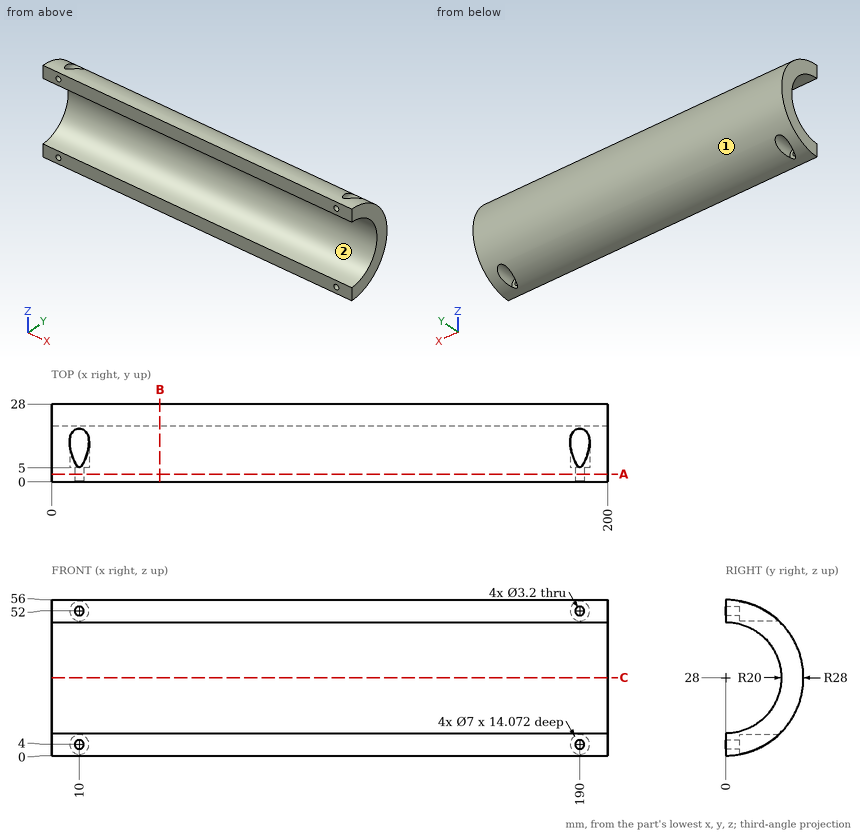
Answer from the drawing. Dimensions are ordinates in mm from the lowest x, y and z of the part. Give positions to 0.01 mm unless a question says otherwise; leave off trailing zeros. Loops run counter-clockwise (first coordinate to the right, second up) from the corner with the lowest first, then second, coordinate; pieces in that order, holes last. Notation, with made-up numbers: (9.25, 17) - (58.25, 17) arc R22 ccw to (58.25, 37) - close; hole circle Ø7 at (37.5, 2.25). An arc over 180 degrees is marked (long way). Answer as a JSON object with one key per item and string values.
1. Flat-ended cylindrical pins translate along their axes: pin 1 Ø2 at (x, z) = (11, 53) entering from +Y; pin 2 Ø11 at (x, z) = (190, 4) entering from +Y; pin 3 Ø1 at (x, z) = (102.5, 21.5) entering from +Y. Find the tip coordinate at first contact, or state that the pin passes through.
Determined:
{"pin 1": "y = 5", "pin 2": "y = 21.02", "pin 3": "y = 27.35"}
2. A cutting plane is placed at B-B (x = 39). Write down the section's boundary in (y, z).
Determined:
{"outline": "(0, 0) arc R28 ccw to (0, 56) - (0, 48) arc R20 cw to (0, 8) - close"}
3. A cutting plane is placed at A-A (y = 2.75). Write down the section's boundary in (x, z) (1 decimal), then the cut area to 3 significant figures.
Determined:
{"outline": "(0, 0.1) - (200, 0.1) - (200, 8.2) - (0, 8.2) - close; (0, 47.8) - (200, 47.8) - (200, 55.9) - (0, 55.9) - close; hole circle Ø3.2 at (10, 4); hole circle Ø3.2 at (10, 52); hole circle Ø3.2 at (190, 4); hole circle Ø3.2 at (190, 52)", "area": "3,190 mm²"}
4. Find the intervals of material crossed by L1, parallel to X at y = 13.5, z = 52; L2, parallel to X at y = 1.9, z = 52; L3, parallel to Z at x = 150.5, y = 13, in increasing order. Write a range as [from, to].
Determined:
{"L1": "[0, 6.5], [13.5, 186.5], [193.5, 200]", "L2": "[0, 8.4], [11.6, 188.4], [191.6, 200]", "L3": "[3.2, 12.8], [43.2, 52.8]"}
5. A cutting plane is placed at C-C (z = 28). Write down the section's boundary in (x, y), then the cut area to 3 significant figures.
Determined:
{"outline": "(0, 20) - (200, 20) - (200, 28) - (0, 28) - close", "area": "1,600 mm²"}
6. For a pull along Z with two mould halves and no side action, classify the marked faces 1 and 2 as pulls with the +Z half, pulls with the -Z half, needs draft (parallel to the pull), parting line crosses it, or undercut.
Determined:
{"face 1": "parting line crosses it", "face 2": "undercut"}
